Autodesk Inventor part; units mm, degrees
ref_plane "YZ Plane" through (0, 0, 0) normal (1, 0, 0) x (0, 1, 0)
ref_plane "XZ Plane" through (0, 0, 0) normal (0, 1, 0) x (-1, 0, 0)
ref_plane "XY Plane" through (0, 0, 0) normal (0, 0, 1) x (1, 0, 0)
sketch "Náčrt1" plane through (0, 0, 0) normal (0, 0, 1) x (1, 0, 0)
  line L0 (30, -47.5) -> (-30, -47.5)
  line L1 (-30, -47.5) -> (-30, 47.5)
  line L2 (-30, 47.5) -> (30, 47.5)
  line L3 (30, 47.5) -> (30, -47.5)
  line L4 (30, -47.5) -> (-30, 47.5) construction
  line L5 (-30, -47.5) -> (30, 47.5) construction
  line L6 (-11.5, -37.5) -> (11.5, -37.5)
  line L7 (11.5, -37.5) -> (11.5, 37.5)
  line L8 (11.5, 37.5) -> (-11.5, 37.5)
  line L9 (-11.5, 37.5) -> (-11.5, -37.5)
  line L10 (-11.5, -37.5) -> (11.5, 37.5) construction
  line L11 (11.5, -37.5) -> (-11.5, 37.5) construction
  line L12 (0, 66.5) -> (0, -66.5)
  line L13 (-42, 0) -> (42, 0)
  point P0 (0, 0)
  point P1 (0, 0)
  dimension "d25" = 60
  dimension "d26" = 95
  dimension "d27" = 23
  dimension "d56" = 10
extrude "Vysunutí1" add sketch "Náčrt1" along normal mid plane 10 contours L0 L12 L6 L7 L13 L3 | L0 L1 L13 L9 L6 L12 | L13 L7 L8 L12 L2 L3 | L1 L2 L12 L8 L9 L13
sketch "Náčrt2" plane through (-30, 47.5, 5) normal (0, 1, 0) x (1, 0, 0)
  point P0 (5, 5)
  point P1 (55, 5)
hole "Díra1" at (-25, 47.5, 0) at (25, 47.5, 0) direction (0, -1, 0) diameter 6 end through all
fillet "Zaoblení1" radius 2 4 edges at (-30, 0, 5) (-30, 0, -5) (30, 0, -5) (30, 0, 5)
sketch "Náčrt3" plane through (0, 0, 5) normal (0, 0, 1) x (1, 0, 0)
  line L0 (11.5, 37.5) -> (11.5, -37.5)
  line L1 (11.5, 17.5) -> (16.5, 17.5)
  line L2 (16.5, 17.5) -> (16.5, 20)
  line L3 (16.5, 20) -> (11.5, 20)
  line L4 (11.5, 20) -> (11.5, 17.5)
  line L5 (-42, 0) -> (42, 0)
  line L6 (0, 66.5) -> (0, -66.5)
  line L7 (-11.5, 37.5) -> (11.5, 37.5)
  line L8 (28, 47.5) -> (-28, 47.5)
  line L9 (-11.5, 17.5) -> (-16.5, 17.5)
  line L10 (-16.5, 17.5) -> (-16.5, 20)
  line L11 (-16.5, 20) -> (-11.5, 20)
  line L12 (-11.5, 20) -> (-11.5, 17.5)
  point P0 (0, 0)
  point P1 (14, 20)
  point P2 (-14, 20)
  dimension "d47" = 5
  dimension "d48" = 2.5
  dimension "d50" = 27.5
extrude "Vysunutí3" cut sketch "Náčrt3" against normal blind 27.5 contours L3 L2 L1 L0 | L9 L10 L11 L12
sketch "Náčrt4" plane through (0, 0, 5) normal (0, 0, 1) x (1, 0, 0)
  line L0 (30, -47.5) -> (28, -47.5)
  line L1 (-30, 47.5) -> (-30, -47.5)
  line L2 (30, -47.5) -> (-30, -47.5)
  line L3 (-30, -47.5) -> (-30, 2.5)
  line L4 (-30, 2.5) -> (30, 2.5)
  line L5 (30, 2.5) -> (30, -47.5)
  point P0 (0, 0)
  dimension "d53" = 50
extrude "Vysunutí4" cut sketch "Náčrt4" against normal blind 10
equation "\"d51\" = d50"
properties part number "SERVO držák"
Input: part model. Units: mm. Frame: model coordinates. A direction names the side the tool comes from. Round coordinates to 2 decimals unless told otherwise and drop trailing zeros. Write each loop counter-clockwise with the first axis right and the second up, starting at its lowest first coordinate (ties: lowest second). Pieces come first, ordered by that corner, then holes. Notation, with made-up numbers: (-32.75, -12.5) - (10.25, -12.5) arc R14 ccw to (10.25, 11.5) - close; hole circle Ø9 at (33.5, -25). An arc over 180 degrees is marked (long way). Write item = value, one per line.
(1) Section query A-A on y = 32. Output: boundary loops of the cut face in (x, z), then the cut area to 3 significant figures.
Geometry check:
outline = (-30, -3) arc R2 ccw to (-28, -5) - (-11.5, -5) - (-11.5, 5) - (-28, 5) arc R2 ccw to (-30, 3) - close; (11.5, -5) - (28, -5) arc R2 ccw to (30, -3) - (30, 3) arc R2 ccw to (28, 5) - (11.5, 5) - close; hole circle Ø6 at (-25, 0); hole circle Ø6 at (25, 0)
area = 310 mm^2
(2) Section query B-B on z = 0. Output: boundary loops of the cut face in (x, y).
Geometry check:
outline = (-30, 2.5) - (-28, 2.5) - (-28, 47.5) - (-30, 47.5) - close; (-22, 2.5) - (-11.5, 2.5) - (-11.5, 17.5) - (-16.5, 17.5) - (-16.5, 20) - (-11.5, 20) - (-11.5, 37.5) - (11.5, 37.5) - (11.5, 20) - (16.5, 20) - (16.5, 17.5) - (11.5, 17.5) - (11.5, 2.5) - (22, 2.5) - (22, 47.5) - (-22, 47.5) - close; (28, 2.5) - (30, 2.5) - (30, 47.5) - (28, 47.5) - close
(3) Material intervals for probe 1 along X at (y, z) = (33, 0); probe 2 along Z at (x, y) = (25, 23.5); probe 3 along X at (y, z) = (35, 2.25), sorted ascending.
Geometry check:
probe_1 = -30 to -28, -22 to -11.5, 11.5 to 22, 28 to 30
probe_2 = -5 to -3, 3 to 5
probe_3 = -30 to -26.98, -23.02 to -11.5, 11.5 to 23.02, 26.98 to 30
(4) Pull-direction query (Y, two-part tool) for faces 4 (the flat face through (-16.5, 19, 0)), 5 (the flat face through (21, 2.5, 0)), 6 (the cylindrical face through (27.93, 24.68, -0.65)); classes: +Y half, -Y half, draft (parallel to the pull), parting line (faces both ways), or undercut.
Geometry check:
face_4 = undercut
face_5 = -Y half
face_6 = draft
(5) Section query D-D on y = 44. Output: boundary loops of the cut face in (x, z).
Geometry check:
outline = (-30, -3) arc R2 ccw to (-28, -5) - (28, -5) arc R2 ccw to (30, -3) - (30, 3) arc R2 ccw to (28, 5) - (-28, 5) arc R2 ccw to (-30, 3) - close; hole circle Ø6 at (-25, 0); hole circle Ø6 at (25, 0)
(6) Section query C-C on x = -25. Output: boundary loops of the cut face in (y, z), then the cut area to 3 significant figures.
Geometry check:
outline = (2.5, -5) - (47.5, -5) - (47.5, -3) - (2.5, -3) - close; (2.5, 3) - (47.5, 3) - (47.5, 5) - (2.5, 5) - close
area = 180 mm^2
(7) Access query for faces 1 (the flat face through (-11.5, 29, 0)), 2 (the flat face through (0, 47.5, 0)), 3 (the flat face through (14, 20, 0)). Directions: +Z, -Z, +X, -X, +Y, -Y. A direction counts if a zero-diameter tool reaches every point of the face in a straight line with its end or side. Return the directions, or none.
Geometry check:
face_1 = +Z, -Z, -Y
face_2 = +Z, -Z, +X, -X, +Y
face_3 = +Z, -Z
(8) Contact query for flat-ended pins moving along their axis: pin 1 Ø12 at (x, y) = (2.5, 17.5) entering from +Z; pin 2 Ø1 at (x, z) = (-4.5, 2.5) entering from -Y. Output: stop coordinate, or through.
Geometry check:
pin_1 = through
pin_2 = 37.5
